Geometry check sheet. Reference: the model listing, model coordinates, mm. Give positions to 0.01 mm unless a question says otherwise; leave off trailing zeros. Order: outer loops, then holes, each group sorted by start corner. A loop starts at its lowest first (then second) coordinate and runs counter-clockwise, first axis right, second up. Notation, with made-up numbers: M -29.5,43.5 L -21.5,43.5 A16 cw -21.5,71.5 Z; hole C -2.75,13 d7. An arc over 180 degrees is marked long. Put each result on its own line as item: value. Start each with the question number.
Q1. Mould release check, pull along Z, two halves, no side actions. Record for faces 1 (the cylindrical face through (40.188, 1.61, -24.062)), 2 (the flat face through (150, 0, -32)): +Z half, -Z half, draft (parallel to the pull), parting line (faces both ways), or undercut.
Q2. Material ranges on L1, parallel to Z at x = 203.2, y = 2.45; L2, parallel to Z at x = 179, y = 1.2; L3, parallel to X at y = 2.75, z = -12.5, recorded low to high.
Q3. Section check A-A on z = -59. Record the cut outline in (x, y) (3 decimals), then the cut area to 3 significant figures.
Q4. Section check B-B on y = 1.9. State how many separate pieces and enclosed holes the cut face has, then the cut area to 3 significant figures.
```python
from build123d import *

# Parameters (mm, degrees)
SKETCH1_W           = 254
SKETCH1_H           = 38.1
SKETCH1_R           = 2.4892
BOSS_EXTRUDE1_DEPTH = 3.175
SKETCH3_R           = 2.4892
SKETCH3_R_2         = 14.2875
CUT_EXTRUDE1_DEPTH  = 312.36051552
FILLET1_R           = 12.7


with BuildPart() as part:
    # Sketch1 → Boss-Extrude1 (new body)
    # profile 1 of 2: a face of its own
    with BuildSketch(Plane(origin=(0, 0, 0), x_dir=(1, 0, 0), z_dir=(0, 1, 0))):
        with Locations((152.4, 19.05)):
            Rectangle(SKETCH1_W, SKETCH1_H)
    # profile 2 of 2: a face of its own
    with BuildSketch(Plane(origin=(0, 0, 0), x_dir=(1, 0, 0), z_dir=(0, 1, 0))):
        Polygon((0, 63.5), (0, 0), (25.4, 0), (25.4, 38.1), (279.4, 38.1), (279.4, 0), (304.8, 0), (304.8, 63.5), align=None)
        with Locations(Location((12.7, 12.7, 0), (0, 0, 270))):
            Circle(SKETCH1_R, mode=Mode.SUBTRACT)
        with Locations(Location((12.7, 25.4, 0), (0, 0, 270))):
            Circle(SKETCH1_R, mode=Mode.SUBTRACT)
        with Locations(Location((292.1, 12.7, 0), (0, 0, 270))):
            Circle(SKETCH1_R, mode=Mode.SUBTRACT)
        with Locations(Location((292.1, 25.4, 0), (0, 0, 270))):
            Circle(SKETCH1_R, mode=Mode.SUBTRACT)
        with Locations(Location((12.7, 38.1, 0), (0, 0, 270))):
            Circle(SKETCH1_R, mode=Mode.SUBTRACT)
        with Locations(Location((12.7, 50.8, 0), (0, 0, 270))):
            Circle(SKETCH1_R, mode=Mode.SUBTRACT)
        with Locations(Location((25.4, 50.8, 0), (0, 0, 270))):
            Circle(SKETCH1_R, mode=Mode.SUBTRACT)
        with Locations(Location((38.1, 50.8, 0), (0, 0, 270))):
            Circle(SKETCH1_R, mode=Mode.SUBTRACT)
        with Locations(Location((50.8, 50.8, 0), (0, 0, 270))):
            Circle(SKETCH1_R, mode=Mode.SUBTRACT)
        with Locations(Location((63.5, 50.8, 0), (0, 0, 270))):
            Circle(SKETCH1_R, mode=Mode.SUBTRACT)
        with Locations(Location((76.2, 50.8, 0), (0, 0, 270))):
            Circle(SKETCH1_R, mode=Mode.SUBTRACT)
        with Locations(Location((88.9, 50.8, 0), (0, 0, 270))):
            Circle(SKETCH1_R, mode=Mode.SUBTRACT)
        with Locations(Location((101.6, 50.8, 0), (0, 0, 270))):
            Circle(SKETCH1_R, mode=Mode.SUBTRACT)
        with Locations(Location((114.3, 50.8, 0), (0, 0, 270))):
            Circle(SKETCH1_R, mode=Mode.SUBTRACT)
        with Locations(Location((127, 50.8, 0), (0, 0, 270))):
            Circle(SKETCH1_R, mode=Mode.SUBTRACT)
        with Locations(Location((139.7, 50.8, 0), (0, 0, 270))):
            Circle(SKETCH1_R, mode=Mode.SUBTRACT)
        with Locations(Location((152.4, 50.8, 0), (0, 0, 270))):
            Circle(SKETCH1_R, mode=Mode.SUBTRACT)
        with Locations(Location((292.1, 38.1, 0), (0, 0, 270))):
            Circle(SKETCH1_R, mode=Mode.SUBTRACT)
        with Locations(Location((165.1, 50.8, 0), (0, 0, 270))):
            Circle(SKETCH1_R, mode=Mode.SUBTRACT)
        with Locations(Location((177.8, 50.8, 0), (0, 0, 270))):
            Circle(SKETCH1_R, mode=Mode.SUBTRACT)
        with Locations(Location((190.5, 50.8, 0), (0, 0, 270))):
            Circle(SKETCH1_R, mode=Mode.SUBTRACT)
        with Locations(Location((203.2, 50.8, 0), (0, 0, 270))):
            Circle(SKETCH1_R, mode=Mode.SUBTRACT)
        with Locations(Location((215.9, 50.8, 0), (0, 0, 270))):
            Circle(SKETCH1_R, mode=Mode.SUBTRACT)
        with Locations(Location((228.6, 50.8, 0), (0, 0, 270))):
            Circle(SKETCH1_R, mode=Mode.SUBTRACT)
        with Locations(Location((241.3, 50.8, 0), (0, 0, 270))):
            Circle(SKETCH1_R, mode=Mode.SUBTRACT)
        with Locations(Location((254, 50.8, 0), (0, 0, 270))):
            Circle(SKETCH1_R, mode=Mode.SUBTRACT)
        with Locations(Location((266.7, 50.8, 0), (0, 0, 270))):
            Circle(SKETCH1_R, mode=Mode.SUBTRACT)
        with Locations(Location((279.4, 50.8, 0), (0, 0, 270))):
            Circle(SKETCH1_R, mode=Mode.SUBTRACT)
        with Locations(Location((292.1, 50.8, 0), (0, 0, 270))):
            Circle(SKETCH1_R, mode=Mode.SUBTRACT)
    extrude(amount=BOSS_EXTRUDE1_DEPTH)

    # Sketch3 → Cut-Extrude1 (cut, through all)
    with BuildSketch(Plane(origin=(0, 3.175, 0), x_dir=(1, 0, 0), z_dir=(0, 1, 0))):
        with Locations(Location((126.98924183, 25.4, 0), (0, 0, 270))):
            Circle(SKETCH3_R)
        with Locations(Location((177.78924183, 25.4, 0), (0, 0, 270))):
            Circle(SKETCH3_R_2)
        with Locations(Location((228.58924183, 25.4, 0), (0, 0, 270))):
            Circle(SKETCH3_R)
        with Locations(Location((38.08924183, 25.4, 0), (0, 0, 270))):
            Circle(SKETCH3_R)
        with Locations(Location((152.38924183, 25.4, 0), (0, 0, 270))):
            Circle(SKETCH3_R)
        with Locations(Location((203.18924183, 25.4, 0), (0, 0, 270))):
            Circle(SKETCH3_R)
    extrude(amount=-CUT_EXTRUDE1_DEPTH, mode=Mode.SUBTRACT)

    # Fillet1
    fillet1_edges = [part.edges().sort_by_distance(p)[0] for p in [
        (0, 1.5875, -63.5),
        (304.8, 1.5875, -63.5),
        (304.8, 1.5875, 0),
        (0, 1.5875, 0),
    ]]
    fillet(fillet1_edges, radius=FILLET1_R)


solid = part.part
```
Results found:
1. face 1: undercut
1. face 2: draft
2. L1: z = -63.5 to -53.29, -48.31 to -27.89, -22.91 to 0
2. L2: z = -63.5 to -52.98, -48.62 to -39.64, -11.16 to 0
2. L3: x = 0 to 10.22, 15.18 to 171.65, 183.93 to 289.62, 294.58 to 304.8
3. outline: M 3.002,0 L 301.798,0 L 301.798,3.175 L 3.002,3.175 Z
3. area: 949 mm^2
4. separate pieces: 1
4. enclosed holes: 35
4. area: 17,900 mm^2
